Study the drawing (mm; zero at the part's minimum x, y, z) and answer. A direction names the side the tool comes from. Coordinates: 2 decimals unless noted, no trailing zeros. Order: outer loops, then holes, each group sorted by start corner. A loop starts at its lowest first (then second) coordinate and runs counter-clockwise, first axis right, second up. Notation, with made-up numbers: (-35, 25) - (-1, 25) arc R22 cw to (-1, 47) - close; hole circle Ø9 at (81.25, 15.5). An arc over 180 degrees is marked (long way). Write item = value, one per line.
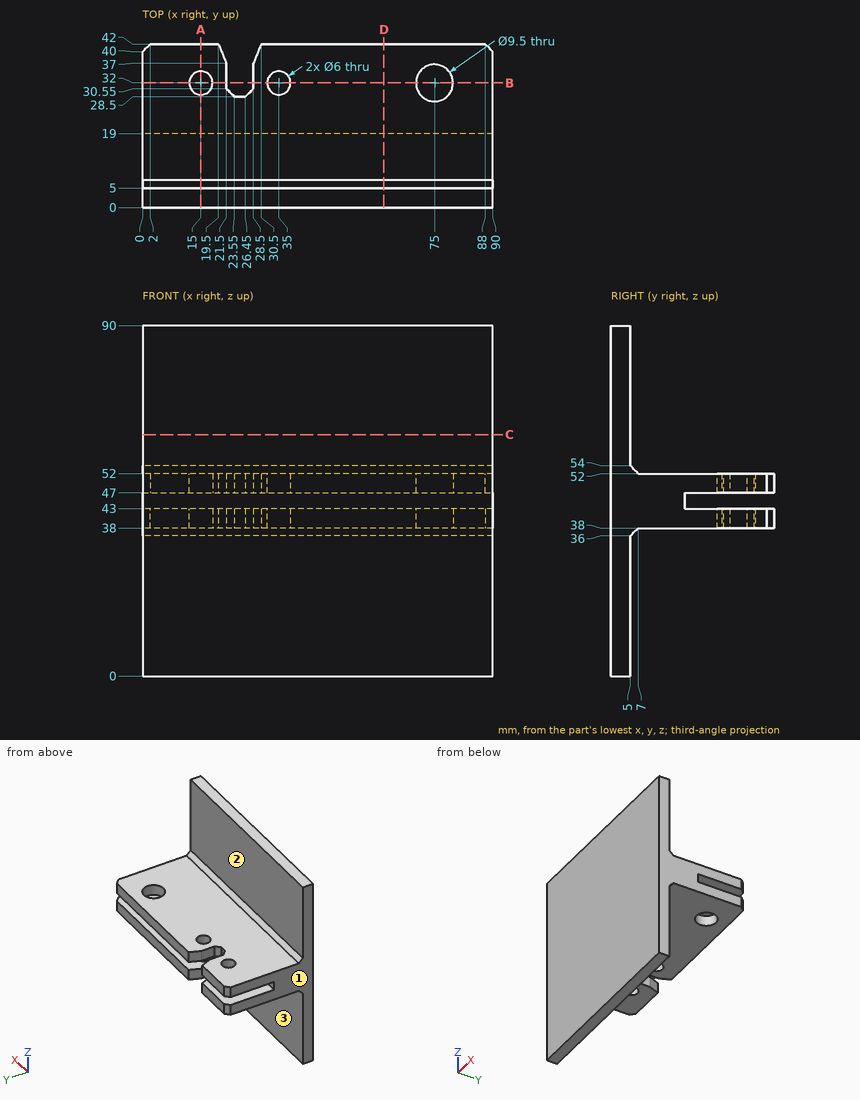
1) The part is cut by section B-B (y = 32). Count the separate pieces of the cut face and the enclosed holes in it, and give its area (3 significant figures).
Returned:
separate_pieces = 10
enclosed_holes = 0
area = 615 mm^2
2) The part is cut by section D-D (x = 62). Determine the outline of the cut face in (y, z), and give its area (3 significant figures).
Returned:
outline = (0, 0) - (5, 0) - (5, 36) - (7, 38) - (42, 38) - (42, 43) - (19, 43) - (19, 47) - (42, 47) - (42, 52) - (7, 52) - (5, 54) - (5, 90) - (0, 90) - close
area = 880 mm^2
3) Straight lines are drawn through the part: line 1 along Z through (x, y) = (12, 34); line 2 along Y through (x, z) = (35, 40.95); line 3 along Z through (x, y) = (55.5, 16). For each, find the intervals that lie inside material, in ascending order. Write a range as from..to.
Returned:
line_1 = 38..43, 47..52
line_2 = 0..29, 35..42
line_3 = 38..52
4) Flat-ended cylindrical pins translate along their axes: pin 1 Ø5.5 at (x, y) = (35, 32) entering from -Z; pin 2 Ø2 at (x, z) = (66.5, 45) entering from +Y; pin 3 Ø8 at (x, y) = (15, 32) entering from +Z; pin 4 Ø2.5 at (x, z) = (25.5, 50) entering from +Y. Find the tip coordinate at first contact, or state that the pin passes through.
Returned:
pin_1 = through
pin_2 = 19
pin_3 = 52
pin_4 = 28.8
5) The part is cut by section A-A (x = 15). Determine the outline of the cut face in (y, z), and give its area (3 significant figures).
Returned:
outline = (0, 0) - (5, 0) - (5, 36) - (7, 38) - (29, 38) - (29, 43) - (19, 43) - (19, 47) - (29, 47) - (29, 52) - (7, 52) - (5, 54) - (5, 90) - (0, 90) - close; (35, 38) - (42, 38) - (42, 43) - (35, 43) - close; (35, 47) - (42, 47) - (42, 52) - (35, 52) - close
area = 820 mm^2
6) For the marked faces 1, 2 and 3, determine the directions among +Z, -Z, +X, -X, +Y, -Y from which every point of the face is accessible in a straight line to the end or side of a thin tool.
Returned:
face_1 = +Z, -Z, -X, +Y, -Y
face_2 = +Z, +X, -X, +Y
face_3 = -Z, +X, -X, +Y
7) The part is cut by section C-C (z = 62). Determine the outline of the cut face in (x, y).
Returned:
outline = (0, 0) - (90, 0) - (90, 5) - (0, 5) - close
